```python
from build123d import *

# Parameters (mm, degrees)
F0_W     = 50
F0_H     = 30
F0_W_2   = 44
F0_H_2   = 24
F1_DEPTH = 162.5
F2_R     = 1.5
F3_R     = 4.5
F4_R     = 3.25
F5_DEPTH = 35
F6_SIZE  = 0.5


with BuildPart() as f1:
    # F0 (on Right) → F1 (new body, symmetric)
    with BuildSketch(Plane.YZ):
        Rectangle(F0_W, F0_H)
        Rectangle(F0_W_2, F0_H_2, mode=Mode.SUBTRACT)
    extrude(amount=F1_DEPTH, both=True)

    # F2
    f2_edges = [f1.edges().sort_by_distance(p)[0] for p in [
        (0, -22, -12),
        (0, -22, 12),
        (0, 22, -12),
        (0, 22, 12),
    ]]
    fillet(f2_edges, radius=F2_R)

    # F3
    f3_edges = [f1.edges().sort_by_distance(p)[0] for p in [
        (0, -25, 15),
        (0, -25, -15),
        (0, 25, -15),
        (0, 25, 15),
    ]]
    fillet(f3_edges, radius=F3_R)

    # F4 (on face) → F5 (cut)
    with BuildSketch(Plane.XY.offset(15)):
        with Locations((-151, 16)):
            Circle(F4_R)
        with Locations((-151, -16)):
            Circle(F4_R)
        with Locations((151, -16)):
            Circle(F4_R)
        with Locations((151, 16)):
            Circle(F4_R)
    extrude(amount=-F5_DEPTH, mode=Mode.SUBTRACT)

    # F6
    f6_edges = [f1.edges().sort_by_distance(p)[0] for p in [
        (-154.25, -16, 15),
        (-154.25, 16, 15),
        (147.75, -16, 15),
        (147.75, 16, 15),
        (147.75, 16, -15),
        (147.75, -16, -15),
        (-154.25, 16, -15),
        (-154.25, -16, -15),
    ]]
    chamfer(f6_edges, length=F6_SIZE)


solid = f1.part
```
Read the model definition and answer for the solid it produces. Units are mm, in the model's axes. Give positions to 0.01 mm unless a question says otherwise; leave off trailing zeros. Write each loop counter-clockwise with the first axis right and the second up, starting at its lowest first coordinate (ties: lowest second). Pieces come first, ordered by that corner, then holes. Notation, with made-up numbers: (-16, -9) -> (4, -9) arc R30 ccw to (4, 22) -> close; hole circle Ø8 at (-6, -12.5). An arc over 180 degrees is marked (long way). Answer in a Markdown table with one row per item.
1) Determine the mould class of faces 1 (the cylindrical face through (-147.9, 16.98, 13.27)), 2 (the flat face through (2, 22, 0)), 3 (the flat face through (2, 0, 12)) for opening direction Z: released by +Z, released by -Z, zero draft, split by the parting line, or undercut.
Results list:
| item | result |
|---|---|
| face 1 | zero draft |
| face 2 | undercut |
| face 3 | undercut |
2) Section C-C on y = 9.5 is taken. Give the vertices of the cut face in (x, z), plus the area to 3 significant figures.
Results list:
| item | result |
|---|---|
| outline | (-162.5, -15) -> (162.5, -15) -> (162.5, -12) -> (-162.5, -12) -> close; (-162.5, 12) -> (162.5, 12) -> (162.5, 15) -> (-162.5, 15) -> close |
| area | 1,950 mm^2 |
3) Straight lines are drawn through the part: line 1 (Y direction, x = -2, z = 0.5); line 2 (Z direction, x = 9, y = -15); line 3 (Y direction, x = 151, z = 14.05). For each, find the intervals that lie inside material, in ascending order. Write a range as [from, to].
Results list:
| item | result |
|---|---|
| line 1 | [-25, -22], [22, 25] |
| line 2 | [-15, -12], [12, 15] |
| line 3 | [-23.27, -19.25], [-12.75, 12.75], [19.25, 23.27] |
4) Section B-B on z = -1 is taken. Give the vertices of the cut face in (x, y), plus the area to 3 significant figures.
Results list:
| item | result |
|---|---|
| outline | (-162.5, -25) -> (162.5, -25) -> (162.5, -22) -> (-162.5, -22) -> close; (-162.5, 22) -> (162.5, 22) -> (162.5, 25) -> (-162.5, 25) -> close |
| area | 1,950 mm^2 |
5) Section A-A on y = -16 is taken. Count the separate pieces of the cut face and the enclosed holes in it, plus the area to 3 significant figures.
Results list:
| item | result |
|---|---|
| separate pieces | 6 |
| enclosed holes | 0 |
| area | 1,870 mm^2 |
6) This flat-tipped pin is pushed along its axis until it touches: pin 1 Ø10 at (x, z) = (-9.5, 11.5) entering from +Y. Where does it stop, or does it pass through?
Results list:
| item | result |
|---|---|
| pin 1 | y = 25 |
